from build123d import *

# Parameters (mm, degrees)
SKETCH_1_R          = 24.9
SKETCH_1_R_2        = 14
EXTRUDE_1_DEPTH     = 7
SKETCH_3_R          = 1.55
CUT_EXTRUDE_2_DEPTH = 10
SKETCH_4_R          = 3.1
CUT_EXTRUDE_3_DEPTH = 1
EXTRUDE_START       = -1
SKETCH_6_R          = 28
SKETCH_6_R_2        = 24.9
EXTRUDE_2_DEPTH     = 1
CUT_EXTRUDE_4_DEPTH = 2.8
FILLET_1_R          = 3


with BuildPart() as part:
    # 草图1 → 凸台-拉伸1 (new body)
    with BuildSketch(Plane.XY):
        Circle(SKETCH_1_R)
        Circle(SKETCH_1_R_2, mode=Mode.SUBTRACT)
    extrude(amount=EXTRUDE_1_DEPTH)

    # 草图3 → 切除-拉伸2 (cut)
    with BuildSketch(Plane(origin=(0, 0, 0), x_dir=(-1, 0, 0), z_dir=(0, 0, -1))):
        with Locations((8.5, -14.722431864)):
            Circle(SKETCH_3_R)
        with Locations((-8.5, -14.722431864)):
            Circle(SKETCH_3_R)
        with Locations((-17, 0)):
            Circle(SKETCH_3_R)
        with Locations((-8.5, 14.722431864)):
            Circle(SKETCH_3_R)
        with Locations((17, 0)):
            Circle(SKETCH_3_R)
        with Locations((8.5, 14.722431864)):
            Circle(SKETCH_3_R)
    extrude(amount=-CUT_EXTRUDE_2_DEPTH, mode=Mode.SUBTRACT)

    # 草图4 → 切除-拉伸3 (cut)
    with BuildSketch(Plane.XY.offset(7)):
        with Locations((17, 0)):
            Circle(SKETCH_4_R)
        with Locations((8.5, -14.722431864)):
            Circle(SKETCH_4_R)
        with Locations((-8.5, -14.722431864)):
            Circle(SKETCH_4_R)
        with Locations((-17, 0)):
            Circle(SKETCH_4_R)
        with Locations((-8.5, 14.722431864)):
            Circle(SKETCH_4_R)
        with Locations((8.5, 14.722431864)):
            Circle(SKETCH_4_R)
    extrude(amount=-CUT_EXTRUDE_3_DEPTH, mode=Mode.SUBTRACT)

    # 草图6 → 凸台-拉伸2 (add)
    with BuildSketch(Plane.XY.offset(7).offset(EXTRUDE_START)):
        Circle(SKETCH_6_R)
        Circle(SKETCH_6_R_2, mode=Mode.SUBTRACT)
    extrude(amount=EXTRUDE_2_DEPTH)

    # 草图7 → 切除-拉伸4 (cut)
    with BuildSketch(Plane(origin=(0, 0, 0), x_dir=(-1, 0, 0), z_dir=(0, 0, -1))):
        Polygon((8.575410724, -17.896962783), (11.286929783, -16.244389721), (11.211519059, -13.069858802), (8.424589276, -11.547900945), (5.713070217, -13.200474007), (5.788480941, -16.375004926), align=None)
        Polygon((19.786929783, -1.521957857), (19.711519059, 1.652573062), (16.924589276, 3.174530919), (14.213070217, 1.521957857), (14.288480941, -1.652573062), (17.075410724, -3.174530919), align=None)
        Polygon((-11.211519059, -16.375004926), (-8.424589276, -17.896962783), (-5.713070217, -16.244389721), (-5.788480941, -13.069858802), (-8.575410724, -11.547900945), (-11.286929783, -13.200474007), align=None)
        Polygon((-19.786929783, 1.521957857), (-19.711519059, -1.652573062), (-16.924589276, -3.174530919), (-14.213070217, -1.521957857), (-14.288480941, 1.652573062), (-17.075410724, 3.174530919), align=None)
        Polygon((-8.575410724, 17.896962783), (-11.286929783, 16.244389721), (-11.211519059, 13.069858802), (-8.424589276, 11.547900945), (-5.713070217, 13.200474007), (-5.788480941, 16.375004926), align=None)
        Polygon((11.211519059, 16.375004926), (8.424589276, 17.896962783), (5.713070217, 16.244389721), (5.788480941, 13.069858802), (8.575410724, 11.547900945), (11.286929783, 13.200474007), align=None)
    extrude(amount=-CUT_EXTRUDE_4_DEPTH, mode=Mode.SUBTRACT)

    # 圆角1
    # the kernel refuses this fillet: 3 mm, written as the material it takes off along each edge
    with BuildSketch(Plane(origin=(0, 0, 0), x_dir=(1, 0, 0), z_dir=(0, -1, 0))) as fillet_1_piece_1:
        with BuildLine():
            CenterArc((14 + FILLET_1_R, FILLET_1_R), FILLET_1_R, 180, 90)
            Line((14, FILLET_1_R), (14, 0))
            Line((14, 0), (14 + FILLET_1_R, 0))
        make_face()
    revolve(axis=Axis((0, 0, 0), (0, 0, 1)), mode=Mode.SUBTRACT)


solid = part.part
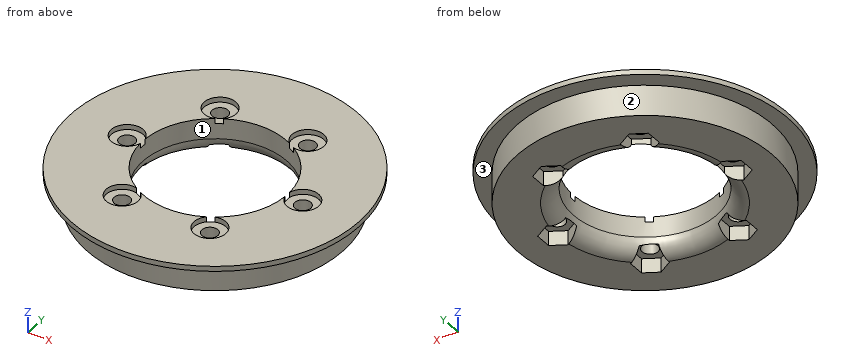
Could you check a few things on this model? Use its own coordinates, in mm. Face numbers are marked on the shaded views. Give positions to 0.01 mm unless a question says otherwise; leave off trailing zeros. Order: outer loops, then holes, each group sorted by start corner. A loop starts at its lowest first (then second) coordinate and runs counter-clockwise, first axis right, second up.
Item 1: I'm going to push flat-ended pins straight in: pin 1 (3.5 mm diameter, centred on x = -8.5, y = 14.72, fed in from +Z); pin 2 (3 mm diameter, centred on x = -8, y = 14.5, fed in from -Z); pin 3 (1 mm diameter, centred on y = -19.5, z = 4.5, fed in from +X). Where does each tip first touch, or does it pass through?
Item 2: I need wall thicknesses on line 1 (Y direction, x = 0, z = 5.4); line 2 (X direction, y = -2.5, z = 6.75); line 3 (X direction, y = -0.5, z = 4). Which ranges of each line are inside material? Lowest first, please.
Item 3: If we section it at A-A, the plane x = 0: Write out the boundary of the cut face in (y, z), plus the area to 3 significant figures.
Item 4: If we section it at B-B, the plane y = 0: Count the separate pieces of the cut face and the enclosed holes in it, plus the area to 3 significant figures.
Item 5: If we mould it in two halves opening along X, with no side actions, what happens to the marked faces 1, 2 and 3? For each: pulls with the +X half, pulls with the -X half, needs draft (parallel to the pull), parting line crosses it, or undercut.
Item 6: If we section it at C-C, the plane z = 5.25: Write out the boundary of the cut face in (x, y).
Item 7: If we section it at D-D, the plane y = -20.5: Write out the boundary of the cut face in (x, z), plus the area to 3 significant figures.
Values:
1. pin 1: stops at z = 6
1. pin 2: stops at z = 2.8
1. pin 3: stops at x = 16.09
2. line 1: y = -24.9 to -14, 14 to 24.9
2. line 2: x = -27.89 to -18.83, -15.17 to -13.77, 13.77 to 15.17, 18.83 to 27.89
2. line 3: x = -24.89 to -18.47, -15.53 to -13.99, 13.99 to 15.53, 18.47 to 24.89
3. outline: (-28, 6) - (-24.9, 6) - (-24.9, 0) - (-17, 0) arc R3 ccw to (-14, 3) - (-14, 7) - (-28, 7) - close; (14, 3) arc R3 ccw to (17, 0) - (24.9, 0) - (24.9, 6) - (28, 6) - (28, 7) - (14, 7) - close
3. area: 155 mm2
4. separate pieces: 4
4. enclosed holes: 0
4. area: 94.9 mm2
5. face 1: undercut
5. face 2: parting line crosses it
5. face 3: needs draft
6. outline: circle Ø49.8 at (0, 0); hole circle Ø3.1 at (-17, 0); hole circle Ø28 at (0, 0); hole circle Ø3.1 at (-8.5, -14.72); hole circle Ø3.1 at (-8.5, 14.72); hole circle Ø3.1 at (8.5, -14.72); hole circle Ø3.1 at (8.5, 14.72); hole circle Ø3.1 at (17, 0)
7. outline: (-19.07, 6) - (-14.13, 6) - (-14.13, 0) - (14.13, 0) - (14.13, 6) - (19.07, 6) - (19.07, 7) - (-19.07, 7) - close
7. area: 208 mm2
